The figure shows three views and two pictorial views of one solid part (mm, origin at its lowest corner). Answer the questions. Coordinates: 2 decimals unless noted, no trailing zeros. Write each loop counter-clockwise with the first axis right and the second up, starting at its lowest first coordinate (ties: lowest second). Pieces come first, ordered by that corner, then holes. Notation, with made-up numbers: M 16.25,85.5 L 67.25,85.5 A16 cw 67.25,98.5 Z; hole C 11.25,-25 d8. An arc over 180 degrees is marked long. Write item = value, one per line.
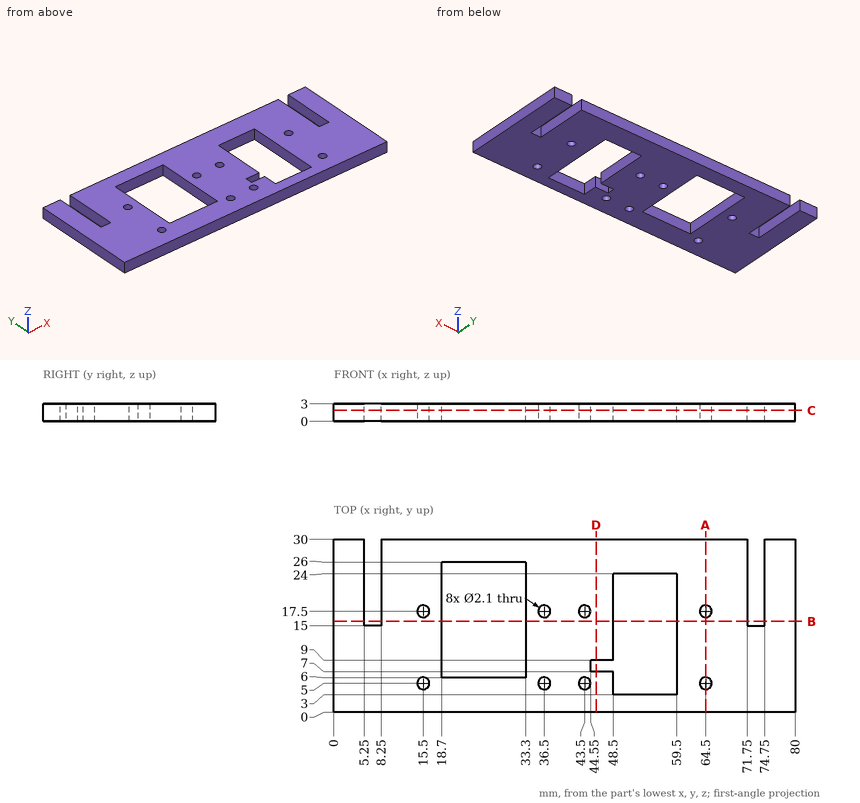
Item 1: Consider line 1 along Y through (x, z) = (43.5, 2.15); line 2 along X through (y, z) = (13, 2.05); line 3 along X through (y, z) = (20.75, 1.75). Determine where each line is inside the solid, lowest interval first. Write a range as from..to.
Worked answers:
line_1 = 0..3.95, 6.05..16.45, 18.55..30
line_2 = 0..18.7, 33.3..48.5, 59.5..80
line_3 = 0..5.25, 8.25..18.7, 33.3..48.5, 59.5..71.75, 74.75..80
Item 2: Find section A-A (x = 64.5). Determine the outline of the cut face in (y, z).
Worked answers:
outline = M 0,0 L 3.95,0 L 3.95,3 L 0,3 Z; M 6.05,0 L 16.45,0 L 16.45,3 L 6.05,3 Z; M 18.55,0 L 30,0 L 30,3 L 18.55,3 Z
Item 3: Find section C-C (z = 1.9). State how many separate pieces and enclosed holes the cut face has, and give its area (3 significant figures).
Worked answers:
separate_pieces = 1
enclosed_holes = 10
area = 1,750 mm²
Item 4: Find section D-D (x = 45.5). Determine the outline of the cut face in (y, z).
Worked answers:
outline = M 0,0 L 7,0 L 7,3 L 0,3 Z; M 9,0 L 30,0 L 30,3 L 9,3 Z
Item 5: Find section B-B (y = 15.75). Determine the outline of the cut face in (x, z).
Worked answers:
outline = M 0,0 L 5.25,0 L 5.25,3 L 0,3 Z; M 8.25,0 L 18.7,0 L 18.7,3 L 8.25,3 Z; M 33.3,0 L 48.5,0 L 48.5,3 L 33.3,3 Z; M 59.5,0 L 71.75,0 L 71.75,3 L 59.5,3 Z; M 74.75,0 L 80,0 L 80,3 L 74.75,3 Z
